from build123d import *

# Parameters (mm, degrees)
ESBO_O1_W                = 30
ESBO_O1_H                = 5
ESBO_O2_R                = 2.5
RESSALTO_EXTRUS_O1_DEPTH = 5


with BuildPart() as part:
    # Esboço1 → Revolução1 (revolve)
    with BuildSketch(Plane.XY):
        with Locations((15, 2.5)):
            Rectangle(ESBO_O1_W, ESBO_O1_H)
    revolve(axis=Axis((30, 0, 0), (-1, 0, 0)))

    # Esboço2 → Ressalto-extrusão1 (add)
    with BuildSketch(Plane(origin=(0, 0, 0), x_dir=(0, 0, -1), z_dir=(1, 0, 0))):
        with BuildLine():
            Line((-37.5, 6), (37.5, 6))
            ThreePointArc((37.5, 6), (43.5, 0), (37.5, -6))
            Line((37.5, -6), (-37.5, -6))
            ThreePointArc((-37.5, -6), (-43.5, 0), (-37.5, 6))
        make_face()
        with Locations((-37.5, 0)):
            Circle(ESBO_O2_R, mode=Mode.SUBTRACT)
        with Locations((37.5, 0)):
            Circle(ESBO_O2_R, mode=Mode.SUBTRACT)
    extrude(amount=-RESSALTO_EXTRUS_O1_DEPTH)


solid = part.part
Geometry check sheet. Reference: the model listing, model coordinates, mm. A direction names the side the tool comes from. Round coordinates to 2 decimals unless told otherwise and drop trailing zeros. Loops run counter-clockwise (first coordinate to the right, second up) from the corner with the lowest first, then second, coordinate; pieces in that order, holes last. Notation, with made-up numbers: (63, 59.25) - (96, 59.25) arc R22 ccw to (96, 81.25) - close; hole circle Ø4 at (-0.75, 3). An arc over 180 degrees is marked (long way). One line per question, with ' | ' between items. Start each with the question number.
1. Cross-section at B-B on y = 0. Record the cut outline in (x, z), then the cut area to 3 significant figures.
2. Cross-section at C-C on y = 3.5. Record the cut outline in (x, z), then the cut area to 3 significant figures.
3. Tool access check on faces 1 (the face through (-2.5, 0.1, -43.5)), 2 (the face through (15.21, -1.08, 4.88)). Record the directions out of +Z, -Z, +X, -X, +Y, -Y that give a thin tool (end or side, any length) a straight path to the whole face; none if there is none.
4. Cross-section at D-D on x = 3. Record the cut outline in (y, z).
5. Draft check along Z on faces 3 (the face through (-2.5, -0.1, 43.5)), 4 (the face through (-2.46, -0.96, 35.19)), 5 (the face through (30, 0, 0)). Enter one of: released by +Z, released by -Z, zero draft, split by the parting line, or undercut.
6. Cross-section at A-A on z = 0. Record the cut outline in (x, y).
7. Scan lines: line 1 (Y direction, x = -2.25, z = -37.5); line 2 (X direction, y = -0.75, z = -14); line 3 (Y direction, x = -2, z = -37). Record each from-to range of solid material in increasing order. Write a range as [from, to].
8. Depth check by flat-ended pin: pin 1 (4 mm diameter, centred on x = 25.5, y = -0.5, fed in from -Z); pin 2 (5 mm diameter, centred on x = 4, z = 24.5, fed in from -Y); pin 3 (1.5 mm diameter, centred on y = 0, z = 21.5, fed in from +X). Enter the tip coordinate at first touch or a pass-through.
Taken from the geometry:
1) outline: (-5, -43.5) - (0, -43.5) - (0, -40) - (-5, -40) - close; (-5, -35) - (0, -35) - (0, -5) - (30, -5) - (30, 5) - (0, 5) - (0, 35) - (-5, 35) - close; (-5, 40) - (0, 40) - (0, 43.5) - (-5, 43.5) - close | area: 685 mm²
2) outline: (-5, -42.37) - (0, -42.37) - (0, -3.57) - (30, -3.57) - (30, 3.57) - (0, 3.57) - (0, 42.37) - (-5, 42.37) - close | area: 638 mm²
3) face 1: -Z, +X, -X | face 2: +X
4) outline: circle Ø10 at (0, 0)
5) face 3: released by +Z | face 4: undercut | face 5: zero draft
6) outline: (-5, -6) - (0, -6) - (0, -5) - (30, -5) - (30, 5) - (0, 5) - (0, 6) - (-5, 6) - close
7) line 1: [-6, -2.5], [2.5, 6] | line 2: [-5, 0] | line 3: [-6, -2.45], [2.45, 6]
8) pin 1: z = -5 | pin 2: through | pin 3: x = 0
